from build123d import *

# Parameters (mm, degrees)
F1_DEPTH  = 200
F2_W      = 280
F2_H      = 40
F3_DEPTH  = 60
F4_W      = 280
F4_H      = 40
F5_DEPTH  = 60
F6_R      = 75
F7_DEPTH  = 300
F8_R      = 7.5
F9_DEPTH  = 40
F10_R     = 7.5
F11_DEPTH = 40
F12_R     = 10


with BuildPart() as f1:
    # F0 (on Right) → F1 (new body)
    with BuildSketch(Plane.YZ):
        Polygon((-150, 94), (-150, 0), (130, 0), (130, 164), (50, 244), (0, 244), align=None)
    extrude(amount=F1_DEPTH)

    # F2 (on face) → F3 (join)
    with BuildSketch(Plane.YZ.offset(200)):
        with Locations((-10, 20)):
            Rectangle(F2_W, F2_H)
    extrude(amount=F3_DEPTH)

    # F4 (on face) → F5 (join)
    with BuildSketch(Plane(origin=(0, 0, 0), x_dir=(0, -1, 0), z_dir=(-1, 0, 0))):
        with Locations((10, 20)):
            Rectangle(F4_W, F4_H)
    extrude(amount=F5_DEPTH)

    # F6 (on face) → F7 (cut)
    with BuildSketch(Plane(origin=(0, -122, 122), x_dir=(1, 0, 0), z_dir=(0, -0.707107, 0.707107))):
        with Locations((100, 66.468037)):
            Circle(F6_R)
    extrude(amount=-F7_DEPTH, mode=Mode.SUBTRACT)

    # F8 (on face) → F9 (cut)
    with BuildSketch(Plane.XY.offset(40)):
        with Locations((-30, 60)):
            Circle(F8_R)
        with Locations((-30, -80)):
            Circle(F8_R)
    extrude(amount=-F9_DEPTH, mode=Mode.SUBTRACT)

    # F10 (on face) → F11 (cut)
    with BuildSketch(Plane.XY.offset(40)):
        with Locations((230, 60)):
            Circle(F10_R)
        with Locations((230, -80)):
            Circle(F10_R)
    extrude(amount=-F11_DEPTH, mode=Mode.SUBTRACT)

    # F12
    f12_edges = [f1.edges().sort_by_distance(p)[0] for p in [
        (-60, -150, 20),
        (260, -150, 20),
        (260, 130, 20),
        (-60, 130, 20),
    ]]
    fillet(f12_edges, radius=F12_R)


solid = f1.part
Verification items for the finished model (mm, model axes). A direction names the side the tool comes from. Give positions to 0.01 mm unless a question says otherwise; leave off trailing zeros. Write each loop counter-clockwise with the first axis right and the second up, starting at its lowest first coordinate (ties: lowest second). Pieces come first, ordered by that corner, then holes. Notation, with made-up numbers: M -33.75,-13.5 L 4.25,-13.5 A22 ccw 4.25,2.5 Z; hole C -37.75,74 d9. An arc over 180 degrees is marked long. Put each result on its own line as item: value. Start each with the question number.
1. Set-up check for faces 4 (the face through (102, -39, 0)), 5 (the face through (230, -12, 40)), 6 (the face through (0, 19, 121)): record each of +Z, -Z, +X, -X, +Y, -Y from which the full face is reachable in a straight line by a thin tool's end or side.
2. Section check C-C (y = -80). Give the number of separate pieces and of enclosed holes in the cut face, and give its area (3 significant figures).
3. Section check D-D (x = 62.5). Record the cut outline in (y, z).
4. Draft check along X on faces 1 (the face through (90.236, 48.995, 150.168)), 2 (the face through (-56.99, 127.15, 20.28)), 3 (the face through (99, 91, 203)). Enter one of: +X half, -X half, draft (parallel to the pull), parting line (faces both ways), or undercut.
5. Scan lines: line 1 along Y through (x, z) = (230, 17.5); line 2 along Z through (x, y) = (244, 31); line 3 along X through (y, z) = (-138, 75.5). Record each from-to range of solid material in increasing order. Write a range as [from, to].
6. Section check B-B (x = 159.5). Record the cut outline in (y, z).
7. Section check A-A (x = 230). Record the cut outline in (y, z).
8. Go/stop test with flat-tipped pins: pin 1 Ø9 at (x, y) = (230, -80) entering from +Z; pin 2 Ø3 at (y, z) = (-27, 49.5) entering from -X; pin 3 Ø8 at (x, y) = (89, 9.5) entering from -Z; pin 4 Ø8 at (x, z) = (93, 195) entering from -Y. Record where each tip stops, or that it passes through.
Answer list:
1. face 4: -Z, +X, -X, +Y, -Y
1. face 5: +Z, +X, +Y, -Y
1. face 6: +Z, -X, +Y, -Y
2. separate pieces: 3
2. enclosed holes: 0
2. area: 25,400 mm2
3. outline: M -150,0 L 2.14,0 L -120.93,123.07 L -150,94 Z; M -29.07,214.93 L 130,55.86 L 130,164 L 50,244 L 0,244 Z
4. face 1: undercut
4. face 2: -X half
4. face 3: draft
5. line 1: [-150, -87.5], [-72.5, 52.5], [67.5, 130]
5. line 2: [0, 40]
5. line 3: [0, 200]
6. outline: M -150,0 L 29.43,0 L -107.29,136.71 L -150,94 Z; M -42.71,201.29 L 130,28.57 L 130,164 L 50,244 L 0,244 Z
7. outline: M -150,0 L -87.5,0 L -87.5,40 L -150,40 Z; M -72.5,0 L 52.5,0 L 52.5,40 L -72.5,40 Z; M 67.5,0 L 130,0 L 130,40 L 67.5,40 Z
8. pin 1: through
8. pin 2: x = 0
8. pin 3: z = 185.32
8. pin 4: y = 0.57
